Input: dimensioned drawing with shaded views. Units: mm. Origin: part minimum x, y, z. A direction names the side the tool comes from. Coordinates: 2 decimals unless noted, no trailing zeros. Write each loop counter-clockwise with the first axis right and the second up, starting at its lowest first coordinate (ties: lowest second). Pieces come first, ordered by that corner, then holes. Notation, with made-up numbers: (-35.75, 62.5) - (15.25, 62.5) arc R10 ccw to (15.25, 74.5) - close; hole circle Ø11 at (53, 77). An arc over 180 degrees is marked (long way). One line per question, with ' | ' between items.
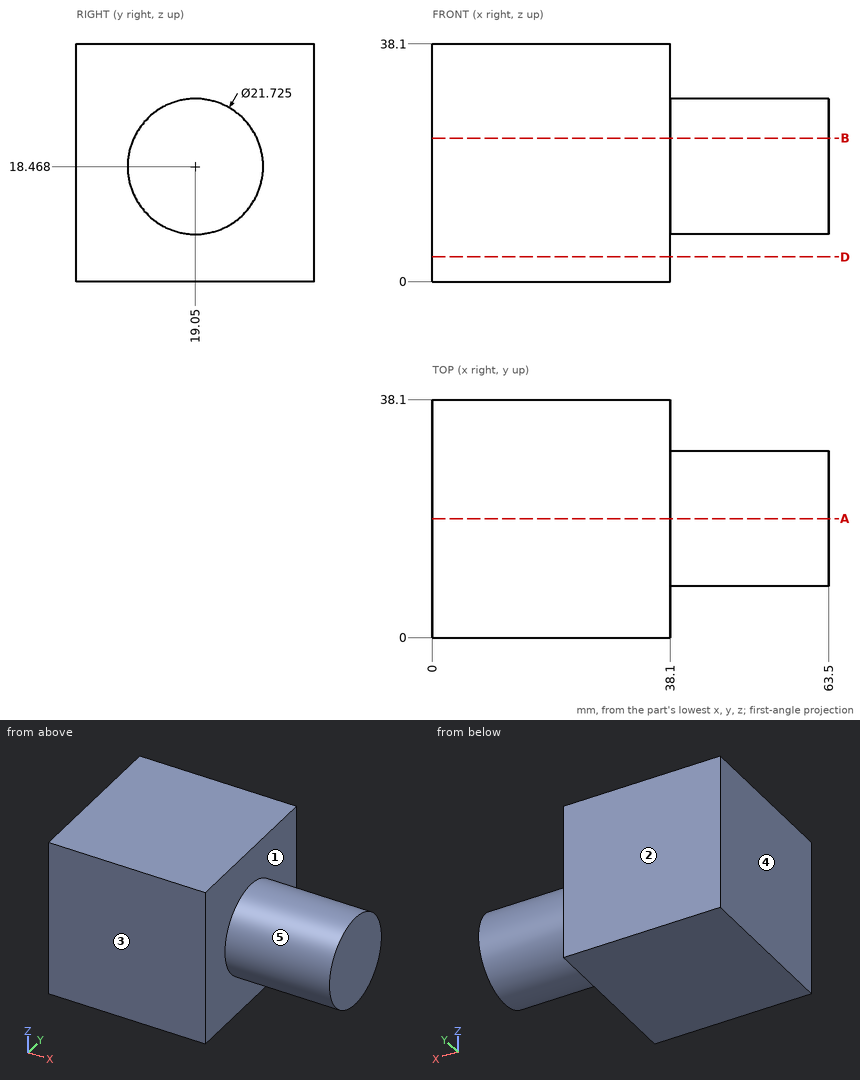
Item 1: Cut plane D-D on z = 4. Return loops of the section in (x, y).
Check sheet entries:
outline: (0, 0) - (38.1, 0) - (38.1, 38.1) - (0, 38.1) - close
Item 2: Pin query (flat end, axial travel): pin 1 Ø3 at (x, z) = (52.5, 12) entering from +Y; pin 2 Ø5 at (x, z) = (55.5, 14) entering from +Y; pin 3 Ø5 at (x, y) = (54, 30.5) entering from +Z. Return the tip coordinate at first contact, or that it passes through.
Check sheet entries:
pin 1: y = 28.71 | pin 2: y = 29.73 | pin 3: z = 24.62
Item 3: Cut plane B-B on z = 23. Return loops of the section in (x, y), and give its area (3 significant figures).
Check sheet entries:
outline: (0, 0) - (38.1, 0) - (38.1, 9.18) - (63.5, 9.18) - (63.5, 28.92) - (38.1, 28.92) - (38.1, 38.1) - (0, 38.1) - close | area: 1,950 mm²
Item 4: Access query for the marked faces 4 and 5. Directions: +Z, -Z, +X, -X, +Y, -Y. A direction counts if a zero-diameter tool reaches every point of the face in a straight line with its end or side. Return the directions, or none.
Check sheet entries:
face 4: +Z, -Z, -X, +Y, -Y | face 5: +X
Item 5: Cut plane A-A on y = 19.05. Return loops of the section in (x, z), and give its area (3 significant figures).
Check sheet entries:
outline: (0, 0) - (38.1, 0) - (38.1, 7.61) - (63.5, 7.61) - (63.5, 29.33) - (38.1, 29.33) - (38.1, 38.1) - (0, 38.1) - close | area: 2,000 mm²
Item 6: Mould query, pull axis Y, two halves, no side actions, for the marked faces 1, 2 and 3. Classes: pulls with the +Y half, pulls with the -Y half, needs draft (parallel to the pull), parting line crosses it, or undercut.
Check sheet entries:
face 1: needs draft | face 2: pulls with the +Y half | face 3: pulls with the -Y half
Item 7: Ray query, line 1 along X through (y, z) = (30.5, 35); line 2 along Y through (x, z) = (60.5, 27); line 3 along Z through (x, y) = (41, 13.5). Return the intervals inside material, ascending. Write a range as [from, to].
Check sheet entries:
line 1: [0, 38.1] | line 2: [12.33, 25.77] | line 3: [9.13, 27.81]
